Design review of the part built by this model. Coordinates are the model's own, in mm. Face numbers are marked on the shaded views. A direction names the side the tool comes from. Give positions to 0.01 mm unless a question says otherwise; leave off trailing zeros. Order: outer loops, then holes, each group sorted by start corner. A loop starts at its lowest first (then second) coordinate and runs counter-clockwise, first axis right, second up. Notation, with made-up numbers: (45, 82) -> (95, 82) arc R30 cw to (95, 114) -> close; hole circle Ø11 at (8.25, 85.5). An arc over 180 degrees is marked (long way). One line per item, written item: value. Start each with the question number.
1) Consider section C-C (x = -46). State the section outline as (y, z) points, plus the area to 3 significant figures.
2) Tool access review of the marked faces 4, 5 and 6: name each direction out of +Z, -Z, +X, -X, +Y, -Y from which nothing blocks a thin tool from reaching the whole face with its end or side.
3) Consider section D-D (y = 42.5). State the section outline as (x, z) points, plus the area to 3 significant figures.
4) The part is to be moulded in two halves that separate along Y. For the marked faces 1, 2 and 3, say which applies: released by +Y, released by -Y, zero draft, split by the parting line, or undercut.
5) Consider section A-A (y = 30). State the section outline as (x, z) points, plus the area to 3 significant figures.
6) Consider section B-B (z = 6.5). State the section outline as (x, y) points.
7) For pin 1 (5.5 mm diameter, centred on x = -53, y = 37, fed in from +Z); pin 2 (10.5 mm diameter, centred on x = 0, y = 25, fed in from +Z); pin 3 (8 mm diameter, centred on x = -39, z = 12, fed in from +Y), all flat-tipped, find the tip position at first contact; note any pin that passes through.
8) Wall thickness on line 1 along Y through (x, z) = (-30, 5.5); line 2 along Y through (x, z) = (-11, 27); line 3 along Z through (x, y) = (-48, 44.5): over which ranges is each line inside the solid? List them lowest first. Write a range as from..to.
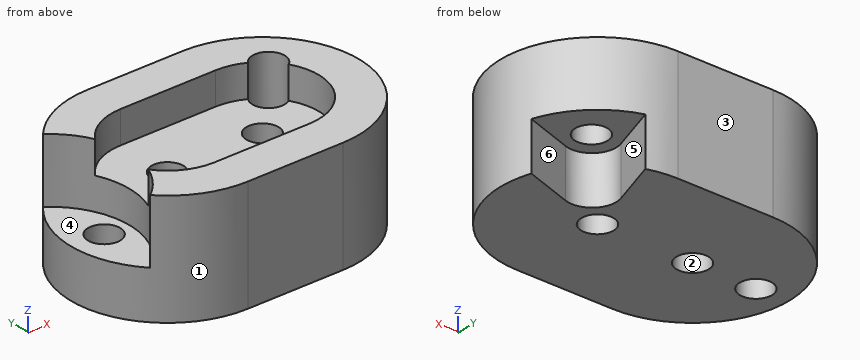
from build123d import *

# Parameters (mm, degrees)
BOSS_EXTRUDE1_DEPTH = 35
CUT_EXTRUDE1_DEPTH  = 10
SKETCH4_R           = 5
CUT_EXTRUDE2_DEPTH  = 113
SKETCH5_R           = 5
CUT_EXTRUDE3_DEPTH  = 20
CUT_EXTRUDE4_DEPTH  = 20
SKETCH7_R           = 5
CUT_EXTRUDE5_DEPTH  = 48
CUT_EXTRUDE7_DEPTH  = 15


with BuildPart() as part:
    # Sketch1 → Boss-Extrude1 (new body)
    with BuildSketch(Plane.XY):
        with BuildLine():
            Line((-30, 60), (0, 60))
            ThreePointArc((0, 60), (30, 30), (0, 0))
            Line((0, 0), (-30, 0))
            ThreePointArc((-30, 0), (-60, 30), (-30, 60))
        make_face()
    extrude(amount=BOSS_EXTRUDE1_DEPTH)

    # Sketch2 → Cut-Extrude1 (cut)
    with BuildSketch(Plane.XY.offset(35)):
        with BuildLine():
            Line((-30, 47.5), (0, 47.5))
            ThreePointArc((0, 47.5), (17.5, 30), (0, 12.5))
            Line((0, 12.5), (-30, 12.5))
            ThreePointArc((-30, 12.5), (-47.5, 30), (-30, 47.5))
        make_face()
    extrude(amount=-CUT_EXTRUDE1_DEPTH, mode=Mode.SUBTRACT)

    # Sketch4 → Cut-Extrude2 (cut)
    with BuildSketch(Plane.XY.offset(25)):
        with Locations((-30, 30)):
            Circle(SKETCH4_R)
        with Locations((0, 30)):
            Circle(SKETCH4_R)
    extrude(amount=-CUT_EXTRUDE2_DEPTH, mode=Mode.SUBTRACT)

    # Sketch5 → Cut-Extrude3 (cut)
    with BuildSketch(Plane.XY.offset(35)):
        with Locations((12.5, 42.5)):
            Circle(SKETCH5_R)
    extrude(amount=-CUT_EXTRUDE3_DEPTH, mode=Mode.SUBTRACT)

    # Sketch6 → Cut-Extrude4 (cut)
    with BuildSketch(Plane.XY.offset(35)):
        with BuildLine():
            ThreePointArc((-52.360679775, 50), (-42.360679775, 30), (-52.360679775, 10))
            ThreePointArc((-52.360679775, 10), (-60, 30), (-52.360679775, 50))
        make_face()
    extrude(amount=-CUT_EXTRUDE4_DEPTH, mode=Mode.SUBTRACT)

    # Sketch7 → Cut-Extrude5 (cut)
    with BuildSketch(Plane.XY.offset(15)):
        with Locations((-50, 30)):
            Circle(SKETCH7_R)
    extrude(amount=-CUT_EXTRUDE5_DEPTH, mode=Mode.SUBTRACT)

    # Sketch8 → Cut-Extrude7 (cut)
    with BuildSketch(Plane(origin=(0, 0, 0), x_dir=(-1, 0, 0), z_dir=(0, 0, -1))):
        with BuildLine():
            Line((-4.099774192, 43.586607173), (-9.099774192, 58.586607173))
            ThreePointArc((-9.099774192, 58.586607173), (-21.213203436, 51.213203436), (-28.586607173, 39.099774192))
            Line((-28.586607173, 39.099774192), (-13.586607173, 34.099774192))
            ThreePointArc((-13.586607173, 34.099774192), (-5.911598069, 35.911598069), (-4.099774192, 43.586607173))
        make_face()
    extrude(amount=-CUT_EXTRUDE7_DEPTH, mode=Mode.SUBTRACT)


solid = part.part
Checked values:
1. outline: (4.62, 0) -> (27, 0) -> (27, 15) -> (17.01, 15) -> (17.01, 35) -> (4.62, 35) -> close; (33, 0) -> (55.38, 0) -> (55.38, 35) -> (42.99, 35) -> (42.99, 15) -> (33, 15) -> close
1. area: 1,170 mm^2
2. face 4: +Z, -X
2. face 5: -Z, +X
2. face 6: -Z, +Y
3. outline: (-57.27, 0) -> (3.83, 0) -> (3.83, 15) -> (7.5, 15) -> (7.5, 25) -> (-42.25, 25) -> (-42.25, 35) -> (-45.71, 35) -> (-45.71, 15) -> (-57.27, 15) -> close; (17.5, 15) -> (27.27, 15) -> (27.27, 35) -> (17.5, 35) -> close
3. area: 1,680 mm^2
4. face 1: split by the parting line
4. face 2: undercut
4. face 3: released by +Y
5. outline: (-60, 0) -> (-55, 0) -> (-55, 15) -> (-60, 15) -> close; (-45, 0) -> (-35, 0) -> (-35, 25) -> (-42.36, 25) -> (-42.36, 15) -> (-45, 15) -> close; (-25, 0) -> (-5, 0) -> (-5, 25) -> (-25, 25) -> close; (5, 0) -> (30, 0) -> (30, 35) -> (17.5, 35) -> (17.5, 25) -> (5, 25) -> close
5. area: 1,550 mm^2
6. outline: (-30, 0) -> (0, 0) arc R30 ccw to (28.59, 39.1) -> (13.59, 34.1) arc R7.5 cw to (4.1, 43.59) -> (9.1, 58.59) arc R30 ccw to (0, 60) -> (-30, 60) arc R30 ccw to start; hole circle Ø10 at (-50, 30); hole circle Ø10 at (-30, 30); hole circle Ø10 at (0, 30)
7. pin 1: stops at z = 15
7. pin 2: stops at z = 25
7. pin 3: stops at y = 59.58
8. line 1: y = 0..25, 35..60
8. line 2: y = 0..12.5, 47.5..60
8. line 3: z = 0..15
